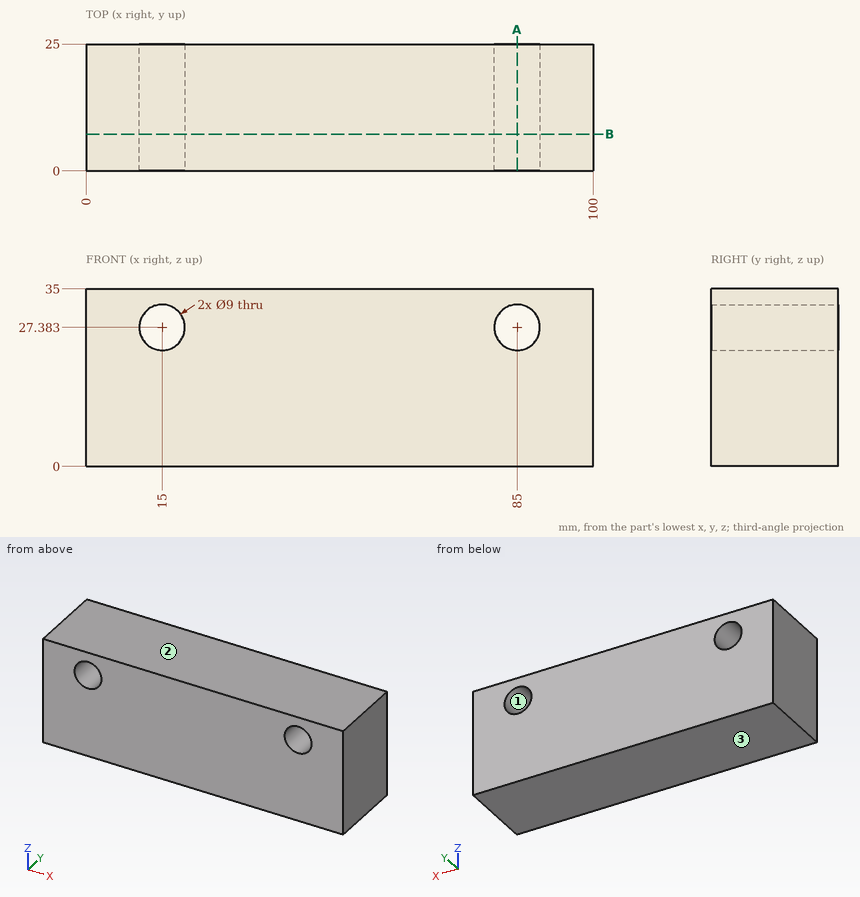
Here's the drawing with two shaded views (mm, measured from the low corner). I have some questions. Round coordinates to 2 decimals unless told otherwise and drop trailing zeros. Loops run counter-clockwise (first coordinate to the right, second up) from the corner with the lowest first, then second, coordinate; pieces in that order, holes last. Notation, with made-up numbers: M 30,9 L 40,9 A30 ccw 40,37 Z; hole C 3,-20.5 d1. An arc over 180 degrees is marked long. Put each result on its own line as item: value.
Q1. I need wall thicknesses on probe 1 along Z at (x, y) = (15, 12); probe 2 along X at (y, z) = (16.5, 24) (1 decimal); probe 3 along X at (y, z) = (4.5, 23.5) (1 decimal). Which ranges of each line are inside material? Lowest first, please.
Check result:
probe 1: 0 to 22.88, 31.88 to 35
probe 2: 0 to 12, 18 to 82, 88 to 100
probe 3: 0 to 12.7, 17.3 to 82.7, 87.3 to 100
Q2. Imagine slicing it at A-A (x = 85). Write out the boundary of the cut face in (y, z).
Check result:
outline: M 0,0 L 25,0 L 25,22.88 L 0,22.88 Z; M 0,31.88 L 25,31.88 L 25,35 L 0,35 Z
Q3. Thinking about a two-plate mould opening in Z: for the marked faces 1, 2 and 3, which applies, released by +Z, released by -Z, zero draft, split by the parting line, or undercut?
Check result:
face 1: undercut
face 2: released by +Z
face 3: released by -Z
Q4. For pin 1 (7 mm diameter, centred on x = 15, z = 27.38, fed in from +Y), with a flat end and sliding along its axis, tell me the tip position at first contact or that it passes through.
Check result:
pin 1: through
Q5. Imagine slicing it at B-B (y = 7.25). Write out the boundary of the cut face in (x, z), then the cut area to 3 significant figures.
Check result:
outline: M 0,0 L 100,0 L 100,35 L 0,35 Z; hole C 15,27.38 d9; hole C 85,27.38 d9
area: 3,370 mm2
